Work out the finished part from the listing and answer in its coordinate system (mm). A direction names the side the tool comes from. Round coordinates to 2 decimals unless told otherwise and drop trailing zeros. Order: outer loops, then holes, each group sorted by start corner. A loop starts at its lowest first (then second) coordinate and runs counter-clockwise, first axis right, second up. Notation, with made-up numbers: (25, 59.5) -> (32, 59.5) arc R27 cw to (32, 84.5) -> close; hole circle Ø11 at (35.5, -21). An arc over 180 degrees is marked (long way). Use a Markdown table: item, result. Add a question column.
Item 1: A cutting plane is placed at A-A, the plane y = -27.5. Determine the outline of the cut face in (x, z), plus the area to 3 significant figures.
Item 2: A tool of negligible diameter and unlimited length cuts with its end or side. For faces 1 (the flat face through (0, -7, -8)), 2 (the cylindrical face through (2.74, 11.7, -3.94)), 3 (the flat face through (0, 0.8, 17)), 4 (the cylindrical face through (-4.9, 49.5, -4.4)), 5 (the flat face through (0, 7, 15)), from which of +Z, -Z, +X, -X, +Y, -Y can it reach the whole face along a straight path? Write none if from no direction.
Item 3: A cutting plane is placed at B-B, the plane z = 4.5. Determine the outline of the cut face in (x, y).
Item 4: A cutting plane is placed at C-C, the plane y = 48.5. Determine the outline of the cut face in (x, z), plus the area to 3 significant figures.
Item 5: For a pull along X with two mould halves and no side action, classify faces 6 (the flat face through (10, 7, 7)), 7 (the cylindrical face through (-4.84, 63.5, -4.44)), 8 (the flat face through (0, -32.5, -4)), 9 (the cylindrical face through (2.4, -11.9, -3.9)) as +X half, -X half, draft (parallel to the pull), parting line (faces both ways), or undercut.
Item 6: A cutting plane is placed at D-D, the plane x = 0. Determine the outline of the cut face in (y, z).
Item 7: Find the intervals of material crossed by L1, parallel to Y at x = -12.5, z = 17; L2, parallel to Z at x = -11.5, y = 41; L3, parallel to Y at x = 0, z = -4, in increasing order. Write a range as [from, to].
Item 8: Flat-ended cylindrical pins translate along their axes: P1, Ø1.3, axis at x = 18, y = 12, coming from the -Z side; P2, Ø2, axis at x = -6, z = 19, coming from the +Y side; P3, Ø8.5, axis at x = 8.5, z = 15, coming from the -Y side. Find the tip coordinate at first contact, or state that the pin passes through.
from build123d import *

# Parameters (mm, degrees)
SKETCH_R             = 1.25
SKETCH_R_2           = 1.6
PAD_DEPTH            = 9
SKETCH002_W          = 55
SKETCH002_H          = 12.7
PAD001_DEPTH         = 28
SKETCH003_W          = 20
SKETCH003_H          = 15
POCKET001_DEPTH      = 63.501
POCKET001_DEPTH_BACK = 32.501
SKETCH001_R          = 5.1
POCKET_DEPTH         = 8


with BuildPart() as part:
    # Sketch → Pad (new body)
    with BuildSketch(Plane.XY):
        with BuildLine():
            Line((-27.5, 32.5), (-12.5, 32.5))
            Line((-12.5, 32.5), (-12.5, 56))
            ThreePointArc((2.5, 56), (-5, 63.5), (-12.5, 56))
            Line((2.5, 56), (2.5, 32.5))
            Line((2.5, 32.5), (27.5, 32.5))
            Line((27.5, 32.5), (27.5, -32.5))
            Line((27.5, -32.5), (-27.5, -32.5))
            Line((-27.5, -32.5), (-27.5, 32.5))
        make_face()
        with Locations((-15, -27.5)):
            Circle(SKETCH_R, mode=Mode.SUBTRACT)
        with Locations((15, -27.5)):
            Circle(SKETCH_R, mode=Mode.SUBTRACT)
        with Locations((-5, 56)):
            Circle(SKETCH_R, mode=Mode.SUBTRACT)
        with Locations((-17.5, 12.5)):
            Circle(SKETCH_R_2, mode=Mode.SUBTRACT)
        with Locations((-17.5, -12.5)):
            Circle(SKETCH_R_2, mode=Mode.SUBTRACT)
        with Locations((17.5, 12.5)):
            Circle(SKETCH_R_2, mode=Mode.SUBTRACT)
        with Locations((17.5, -12.5)):
            Circle(SKETCH_R_2, mode=Mode.SUBTRACT)
        Circle(SKETCH_R_2, mode=Mode.SUBTRACT)
        with Locations((-17.5, 0)):
            Circle(SKETCH_R_2, mode=Mode.SUBTRACT)
        with Locations((17.5, 0)):
            Circle(SKETCH_R_2, mode=Mode.SUBTRACT)
        with BuildLine():
            ThreePointArc((-2.5, 47), (-5, 49.5), (-7.5, 47))
            Line((-7.5, 47), (-7.5, 35))
            ThreePointArc((-7.5, 35), (-5, 32.5), (-2.5, 35))
            Line((-2.5, 47), (-2.5, 35))
        make_face(mode=Mode.SUBTRACT)
    extrude(amount=-PAD_DEPTH)

    # Sketch002 → Pad001 (join)
    with BuildSketch(Plane.XY):
        with Locations((0, 7.15)):
            Rectangle(SKETCH002_W, SKETCH002_H)
    extrude(amount=PAD001_DEPTH)

    # Sketch003 → Pocket001 (cut, two sides)
    with BuildSketch(Plane.XZ) as pocket001_sk:
        with Locations((0, 7.5)):
            Rectangle(SKETCH003_W, SKETCH003_H)
    extrude(amount=-POCKET001_DEPTH, mode=Mode.SUBTRACT)
    extrude(pocket001_sk.sketch, amount=POCKET001_DEPTH_BACK, mode=Mode.SUBTRACT)

    # Sketch001 → Pocket (cut)
    with BuildSketch(Plane.XY):
        with Locations((0, 7.4)):
            Circle(SKETCH001_R)
        with Locations((0, -7.4)):
            Circle(SKETCH001_R)
    extrude(amount=-POCKET_DEPTH, mode=Mode.SUBTRACT)


solid = part.part
Reported:
| question | item | result |
|---|---|---|
| 1 | outline | (-27.5, -9) -> (-16.25, -9) -> (-16.25, 0) -> (-27.5, 0) -> close; (-13.75, -9) -> (13.75, -9) -> (13.75, 0) -> (-13.75, 0) -> close; (16.25, -9) -> (27.5, -9) -> (27.5, 0) -> (16.25, 0) -> close |
| 1 | area | 450 mm² |
| 2 | face 1 | +Z |
| 2 | face 2 | none |
| 2 | face 3 | +Z, +X, -X, -Y |
| 2 | face 4 | +Z, -Z |
| 2 | face 5 | +Y, -Y |
| 3 | outline | (-27.5, 0.8) -> (-10, 0.8) -> (-10, 13.5) -> (-27.5, 13.5) -> close; (10, 0.8) -> (27.5, 0.8) -> (27.5, 13.5) -> (10, 13.5) -> close |
| 4 | outline | (-12.5, -9) -> (-7, -9) -> (-7, 0) -> (-12.5, 0) -> close; (-3, -9) -> (2.5, -9) -> (2.5, 0) -> (-3, 0) -> close |
| 4 | area | 99.0 mm² |
| 5 | face 6 | undercut |
| 5 | face 7 | parting line |
| 5 | face 8 | draft |
| 5 | face 9 | undercut |
| 6 | outline | (-32.5, -9) -> (-1.6, -9) -> (-1.6, 0) -> (-2.3, 0) -> (-2.3, -8) -> (-12.5, -8) -> (-12.5, 0) -> (-32.5, 0) -> close; (0.8, 15) -> (13.5, 15) -> (13.5, 28) -> (0.8, 28) -> close; (1.6, -9) -> (61.59, -9) -> (61.59, 0) -> (12.5, 0) -> (12.5, -8) -> (2.3, -8) -> (2.3, 0) -> (1.6, 0) -> close |
| 7 | L1 | [0.8, 13.5] |
| 7 | L2 | [-9, 0] |
| 7 | L3 | [-32.5, -12.5], [-2.3, -1.6], [1.6, 2.3], [12.5, 61.59] |
| 8 | P1 | z = 0 |
| 8 | P2 | y = 13.5 |
| 8 | P3 | y = 0.8 |
